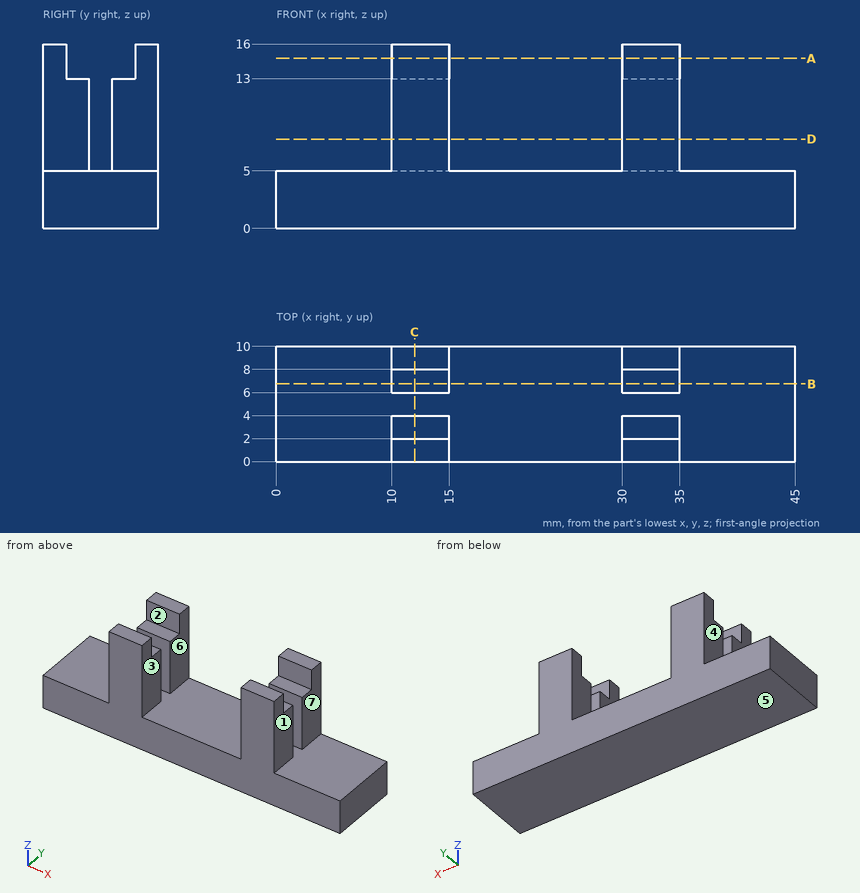
Answer from the drawing. Dimensions are ordinates in mm from the lowest x, y and z of the part. A direction names the side the tool comes from. Round coordinates to 2 decimals unless told otherwise and drop trailing zeros. Order: outer loops, then holes, each group sorted by start corner. A loop starts at its lowest first (then second) coordinate and runs counter-clockwise, first axis right, second up.
1) For the marked faces 1, 2, 3 and 4, determine the directions among +Z, -Z, +X, -X, +Y, -Y from which every point of the face is accessible in a straight line to the end or side of a thin tool.
2) Straight lines are drawn through the part: L1, parallel to X at y = 6.5, z = 10.75; L2, parallel to Z at x = 37.5, y = 5; L3, parallel to Z at x = 33, y = 3. For each, find the intervals that lie inside material, in ascending order.
3) The part is cut by section B-B on y = 6.75. Write down the section's boundary in (x, z).
4) The part is cut by section A-A on z = 14.75. Write down the section's boundary in (x, y), plus the area to 3 significant figures.
5) The part is cut by section D-D on z = 7.75. Write down the section's boundary in (x, y), plus the area to 3 significant figures.
6) Flat-ended cylindrical pins translate along their axes: pin 1 (2 mm diameter, centred on y = 7.5, z = 10.5, fed in from -X); pin 2 (3 mm diameter, centred on x = 14.5, y = 4.5, fed in from +Z); pin 3 (2 mm diameter, centred on y = 7.5, z = 8, fed in from +X). Find the tip coordinate at first contact, or state that the pin passes through.
7) The mould has two halves that part along X. Classify the marked faces 5, 6 and 7: released by +X, released by -X, zero draft, split by the parting line, or undercut.
8) The part is cut by section C-C on x = 12. Write down the section's boundary in (y, z).
Resolved:
1. face 1: +Z, +X, +Y, -Y
1. face 2: +Z, +X, -X
1. face 3: +Z, +Y, -Y
1. face 4: +Z, -X, +Y, -Y
2. L1: x = 10 to 15, 30 to 35
2. L2: z = 0 to 5
2. L3: z = 0 to 13
3. outline: (0, 0) - (45, 0) - (45, 5) - (35, 5) - (35, 13) - (30, 13) - (30, 5) - (15, 5) - (15, 13) - (10, 13) - (10, 5) - (0, 5) - close
4. outline: (10, 0) - (15, 0) - (15, 2) - (10, 2) - close; (10, 8) - (15, 8) - (15, 10) - (10, 10) - close; (30, 0) - (35, 0) - (35, 2) - (30, 2) - close; (30, 8) - (35, 8) - (35, 10) - (30, 10) - close
4. area: 40.0 mm2
5. outline: (10, 0) - (15, 0) - (15, 4) - (10, 4) - close; (10, 6) - (15, 6) - (15, 10) - (10, 10) - close; (30, 0) - (35, 0) - (35, 4) - (30, 4) - close; (30, 6) - (35, 6) - (35, 10) - (30, 10) - close
5. area: 80.0 mm2
6. pin 1: stops at x = 10
6. pin 2: stops at z = 13
6. pin 3: stops at x = 35
7. face 5: zero draft
7. face 6: undercut
7. face 7: released by +X
8. outline: (0, 0) - (10, 0) - (10, 16) - (8, 16) - (8, 13) - (6, 13) - (6, 5) - (4, 5) - (4, 13) - (2, 13) - (2, 16) - (0, 16) - close
